Study the drawing (mm; zero at the part's minimum x, y, z) and answer. A direction names the side the tool comes from. Coordinates: 2 decimals unless noted, no trailing zeros. Order: outer loops, then holes, each group sorted by start corner. A loop starts at its lowest first (then second) coordinate and runs counter-clockwise, first axis right, second up.
1. Find the intervals of material crossed by probe 1 along X at (y, z) = (27.5, 101.5); probe 2 along Z at (x, y) = (14, 29); probe 3 along Y at (x, z) = (16.5, 107), in increasing order.
2. The part is cut by section B-B, the plane z = 134. Give the vertices of the cut face in (x, y).
3. The part is cut by section A-A, the plane y = 65. Give the vertices of the cut face in (x, z), then the cut area to 3 significant figures.
4. Determine the mould class of the marked faces 1, 2 and 3 for opening direction X: +X half, -X half, draft (parallel to the pull), parting line (faces both ways), or undercut.
5. Flat-ended cylindrical pins translate along their axes: pin 1 Ø12 at (x, z) = (54.5, 76.5) entering from +Y; pin 2 Ø6 at (y, z) = (33.5, 138.5) entering from -X; pin 3 Ø4.5 at (x, z) = (66.5, 123) entering from -Y. Find the tip coordinate at first contact, or state that the pin passes through.
6. The part is cut by section D-D, the plane x = 7.5. Give the vertices of the cut face in (y, z).
7. The part is cut by section C-C, the plane y = 17. Give the vertices of the cut face in (x, z), then the cut area to 3 significant figures.
8. A tool of negligible diameter and unlimited length cuts with its end or side. For the marked faces 4, 5, 6, 7 and 8, from which of +Z, -Z, +X, -X, +Y, -Y can it reach the whole face along a straight path? Write none if from no direction.
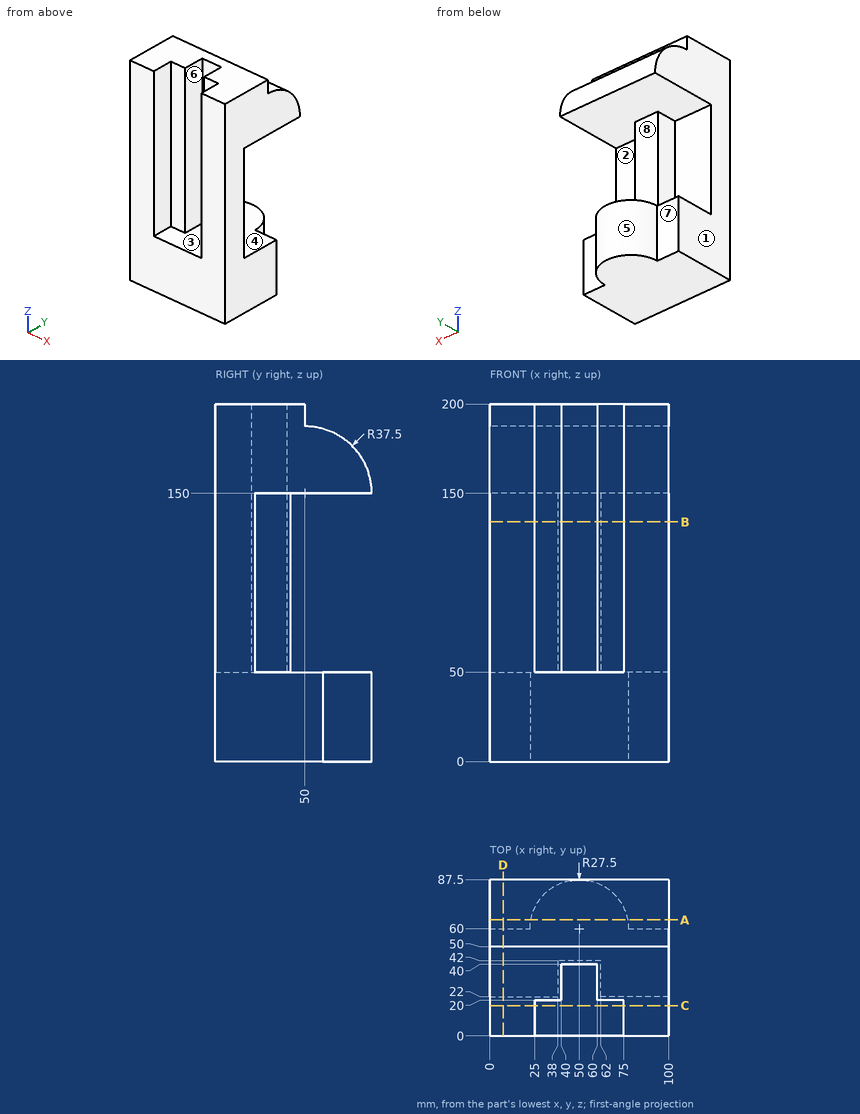
Geometry says:
1. probe 1: x = 38 to 40, 60 to 62
1. probe 2: z = 0 to 50, 150 to 200
1. probe 3: y = 0 to 22
2. outline: (0, 0) - (25, 0) - (25, 20) - (40, 20) - (40, 40) - (60, 40) - (60, 20) - (75, 20) - (75, 0) - (100, 0) - (100, 22) - (62, 22) - (62, 42) - (38, 42) - (38, 22) - (0, 22) - close
3. outline: (0, 150) - (100, 150) - (100, 184.37) - (0, 184.37) - close; (22.96, 0) - (77.04, 0) - (77.04, 50) - (22.96, 50) - close
3. area: 6,140 mm2
4. face 1: -X half
4. face 2: draft
4. face 3: undercut
5. pin 1: stops at y = 42
5. pin 2: stops at x = 38
5. pin 3: stops at y = 20
6. outline: (0, 0) - (60, 0) - (60, 50) - (22, 50) - (22, 150) - (87.5, 150) arc R37.5 ccw to (50, 187.5) - (50, 200) - (0, 200) - close
7. outline: (0, 0) - (100, 0) - (100, 200) - (75, 200) - (75, 50) - (25, 50) - (25, 200) - (0, 200) - close
7. area: 12,500 mm2
8. face 4: +Y
8. face 5: -Z, +Y
8. face 6: +Z, -Y
8. face 7: -Z, -X, +Y
8. face 8: +X, -X, +Y
